from build123d import *

# Parameters (mm, degrees)
F1_DEPTH = 415
F3_D     = 8
F5_D     = 8


with BuildPart() as f1:
    # F0 (on Top) → F1 (new body, symmetric)
    with BuildSketch(Plane.XY):
        Polygon((-20, -20), (20, -20), (20, 20), (16, 20), (16, -16), (-16, -16), (-16, 20), (-20, 20), align=None)
    extrude(amount=F1_DEPTH, both=True)

    # F3 (through all)
    with Locations(Plane.YZ.offset(20)):
        with Locations((-10, 397), (10, 397)):
            Hole(F3_D / 2)

    # F5 (through all)
    with Locations(Plane.XZ.offset(20)):
        with Locations((0, -380), (10.1231555268, -400), (-9.8768444732, -400)):
            Hole(F5_D / 2)


solid = f1.part
Geometry check sheet. Reference: the model listing, model coordinates, mm. A direction names the side the tool comes from. Give positions to 0.01 mm unless a question says otherwise; leave off trailing zeros. Loops run counter-clockwise (first coordinate to the right, second up) from the corner with the lowest first, then second, coordinate; pieces in that order, holes last.
(1) Thickness scan on L1, parallel to Y at x = 16.95, z = 397; L2, parallel to X at y = -6.5, z = 150.5; L3, parallel to Z at x = 18.85, y = 10. Record the ranges inside material, lowest first.
From the geometry:
L1: y = -20 to -14, -6 to 6, 14 to 20
L2: x = -20 to -16, 16 to 20
L3: z = -415 to 393, 401 to 415
(2) Set-up check for faces 1 (the flat face through (16, 2, 6)), 2 (the flat face through (-0.1, -16.2, -415)): record each of +Z, -Z, +X, -X, +Y, -Y from which the full face is reachable in a straight line by a thin tool's end or side.
From the geometry:
face 1: +Z, -Z, +Y
face 2: -Z, +X, -X, +Y, -Y
(3) Section check A-A on z = 249. Record the cut outline in (x, y).
From the geometry:
outline: (-20, -20) - (20, -20) - (20, 20) - (16, 20) - (16, -16) - (-16, -16) - (-16, 20) - (-20, 20) - close
(4) Depth check by flat-ended pin: pin 1 Ø10.5 at (x, z) = (-9.88, -400) entering from +Y. Enter the tip coordinate at first touch or a pass-through.
From the geometry:
pin 1: stops at y = -16
(5) Release check for a two-part mould opening along X. For faces 3 (the flat face through (20, 0, 6)), 4 (the flat face through (0, -16, 6)), 5 (the flat face through (-0.1, -16.2, 415)), 6 (the flat face through (-20, 0, 6)) record: released by +X, released by -X, zero draft, split by the parting line, or undercut.
From the geometry:
face 3: released by +X
face 4: undercut
face 5: zero draft
face 6: released by -X
